Can you work these out from the drawing? Everything is in mm from the part's minimum corner. Coordinates: 2 decimals unless noted, no trailing zeros. Order: outer loops, then holes, each group sorted by start corner. A loop starts at its lowest first (then second) coordinate and runs counter-clockwise, first axis right, second up. Notation, with made-up numbers: (-6.5, 48) -> (28.5, 48) arc R19 ccw to (28.5, 67) -> close; hole circle Ø9 at (12.5, 49). An arc over 180 degrees is marked (long way). Use a Markdown table: item, result. Add a question column.
1) If we section it at C-C (z = 151): Write out the boundary of the cut face in (x, y), plus the area to 3 significant figures.
2) If we section it at A-A (x = 9.4): Write out the boundary of the cut face in (y, z), plus the area to 3 significant figures.
3) Will these pins go through, and if not, where does the flat tip stop? pin 1 Ø1 at (x, y) = (7, 13.5) entering from -Z; pin 2 Ø3 at (y, z) = (13.5, 195.5) entering from +X; pin 3 Ø2 at (x, z) = (7.5, 210.5) entering from +Y.
4) If we section it at D-D (z = 238.5): Write out the boundary of the cut face in (x, y).
5) If I drill on L1, parallel to Z at x = 17, y = 13; L2, parallel to X at y = 9, z = 60; L3, parallel to X at y = 11, z = 97.5, over which ranges is the centre line in solid material (lowest first)? Write a range as [from, to].
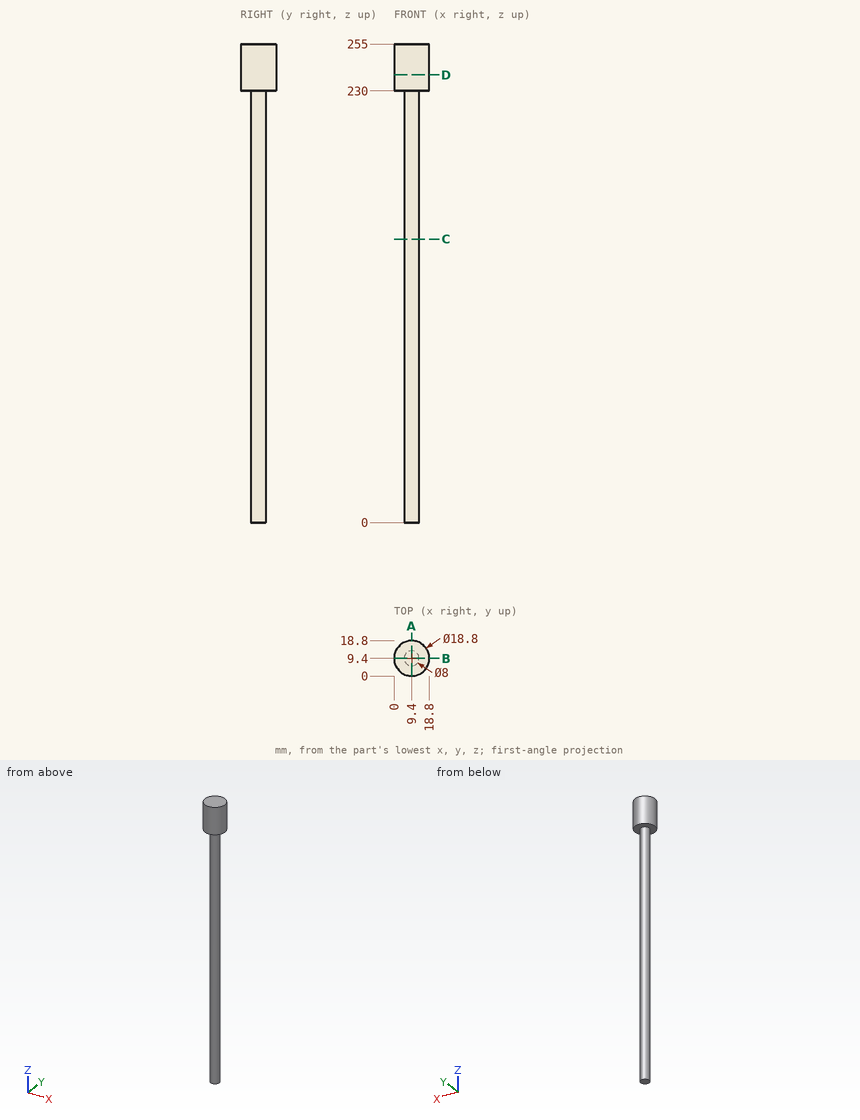
Answer sheet:
| question | item | result |
|---|---|---|
| 1 | outline | circle Ø8 at (9.4, 9.4) |
| 1 | area | 50.3 mm2 |
| 2 | outline | (0, 230) -> (5.4, 230) -> (5.4, 0) -> (13.4, 0) -> (13.4, 230) -> (18.8, 230) -> (18.8, 255) -> (0, 255) -> close |
| 2 | area | 2,310 mm2 |
| 3 | pin 1 | z = 230 |
| 3 | pin 2 | x = 12.44 |
| 3 | pin 3 | y = 13.3 |
| 4 | outline | circle Ø18.8 at (9.4, 9.4) |
| 5 | L1 | [230, 255] |
| 5 | L2 | [5.42, 13.38] |
| 5 | L3 | [5.73, 13.07] |
